For this review, take the finished solid that the model builds, in its own axes (mm). Coordinates: 2 decimals unless noted, no trailing zeros. Write each loop counter-clockwise with the first axis right and the second up, starting at its lowest first coordinate (ties: lowest second). Pieces come first, ordered by that corner, then holes. Notation, with made-up numbers: (60.5, 84) - (78.5, 84) arc R12 cw to (78.5, 90) - close; hole circle Ø11 at (28, 31.5). An arc over 180 degrees is marked (long way). Write each question's results on one line, items separated by ' | '.
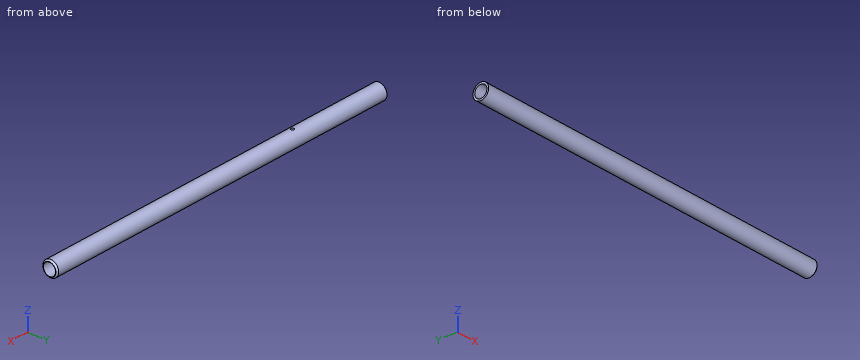
from build123d import *

# Parameters (mm, degrees)
F1_R     = 10.3124
F1_R_2   = 8.0264
F2_DEPTH = 241.3
F4_D     = 3.9624
F4_DEPTH = 12.7
F4_START = 0.1921017
F4_TIP   = 1.1904250584
F5_SIZE  = 1.905


with BuildPart() as f2:
    # F1 (on Right) → F2 (new body, symmetric)
    with BuildSketch(Plane.YZ):
        Circle(F1_R)
        Circle(F1_R_2, mode=Mode.SUBTRACT)
    extrude(amount=F2_DEPTH, both=True)

    # F4
    # its depths count from where the whole tool has entered the part; down to there all is cleared
    with Locations(Plane.XY.offset(10.3124).offset(-F4_START)):
        with Locations((-114.3, 0)):
            Hole(F4_D / 2, depth=F4_DEPTH)
            with Locations((0, 0, -(F4_DEPTH + F4_TIP / 2))):  # 118° drill point
                Cone(0, F4_D / 2, F4_TIP, mode=Mode.SUBTRACT)

    # F5
    f5_edges = [f2.edges().sort_by_distance(p)[0] for p in [
        (241.3, -10.3124, 0),
    ]]
    chamfer(f5_edges, length=F5_SIZE)


solid = f2.part
Q1. For pin 1 (6 mm diameter, centred on x = 136.5, y = -7, fed in from -Z); pin 2 (3 mm diameter, centred on x = -128, y = -3, fed in from +Z); pin 3 (2 mm diameter, centred on x = 187, y = -1.5, fed in from +Z), all flat-tipped, find the tip position at first contact; note any pin that passes through.
Results found:
pin 1: z = -9.51 | pin 2: z = 10.2 | pin 3: z = 10.3
Q2. Take a section at A-A on z = 0. State the section outline as (x, y) points (3 decimals).
Results found:
outline: (-241.3, -10.312) - (239.395, -10.312) - (241.3, -8.407) - (241.3, -8.026) - (-241.3, -8.026) - close; (-241.3, 8.026) - (241.3, 8.026) - (241.3, 8.407) - (239.395, 10.312) - (-241.3, 10.312) - close
Q3. Wall thickness on line 1 along Z through (x, y) = (131, 0); line 2 along Y through (x, z) = (-71.5, 4.75); line 3 along Y through (x, z) = (-220.5, -4.25): over which ranges is each line inside the solid? List them lowest first. Write a range as from..to.
Results found:
line 1: -10.31..-8.03, 8.03..10.31 | line 2: -9.15..-6.47, 6.47..9.15 | line 3: -9.4..-6.81, 6.81..9.4
Q4. Take a section at B-B on x = -192. State the section outline as (y, z) points, plus the area to 3 significant figures.
Results found:
outline: circle Ø20.62 at (0, 0); hole circle Ø16.05 at (0, 0) | area: 132 mm2
